Autodesk Inventor part; units mm, degrees
ref_plane "YZ Plane" through (0, 0, 0) normal (1, 0, 0) x (0, 1, 0)
ref_plane "XZ Plane" through (0, 0, 0) normal (0, 1, 0) x (-1, 0, 0)
ref_plane "XY Plane" through (0, 0, 0) normal (0, 0, 1) x (1, 0, 0)
sketch "Sketch1" plane through (0, 0, 0) normal (0, 0, 1) x (1, 0, 0)
  line L0 (-122.55, 8.89) -> (122.55, 8.89)
  line L1 (122.55, 8.89) -> (122.55, -8.89)
  line L2 (122.55, -8.89) -> (-122.55, -8.89)
  line L3 (-122.55, -8.89) -> (-122.55, 8.89)
  line L4 (-122.55, 8.89) -> (122.55, -8.89) construction
  line L5 (122.55, 8.89) -> (-122.55, -8.89) construction
  point P0 (0, 0)
  dimension "d0" = 245.1
  dimension "d1" = 17.78
extrude "Extrusion1" add sketch "Sketch1" along normal blind 6.2
fillet "Fillet1" radius 8.89 1 edges at (122.55, 8.89, 3.1)
fillet "Fillet2" radius 8.89 1 edges at (122.55, -8.89, 3.1)
fillet "Fillet3" radius 8.89 1 edges at (-122.55, -8.89, 3.1)
fillet "Fillet4" radius 8.89 1 edges at (-122.55, 8.89, 3.1)
sketch "Sketch6" plane through (0, 0, 0) normal (0, 0, -1) x (-1, 0, 0)
  circle A0 centre (111.8854, 0) radius 5.5644
  point P0 (0, 0)
extrude "Extrusion4" add sketch "Sketch6" along normal blind 7.2
sketch "Sketch7" plane through (0, 0, 0) normal (0, 0, -1) x (-1, 0, 0)
  point P0 (0, 0)
  point P1 (-112.5539, 0.8007)
hole "Hole3" at (112.5539, 0.8007, 0) direction (0, 0, 1) diameter 12.4257 end through all
equation "\"BendRadius\" = Thickness"
equation "\"BendReliefWidth\" = Thickness"
equation "\"BendReliefDepth\" = 0.5 * Thickness"
equation "\"CornerReliefSize\" = 4 * Thickness"
equation "\"MinimumRemnant\" = 2 * Thickness"
equation "\"TransitionRadius\" = BendRadius"
equation "\"JacobiRadiusSize\" = BendRadius"
equation "\"GapSize\" = Thickness"
properties part number "cranker rod part"
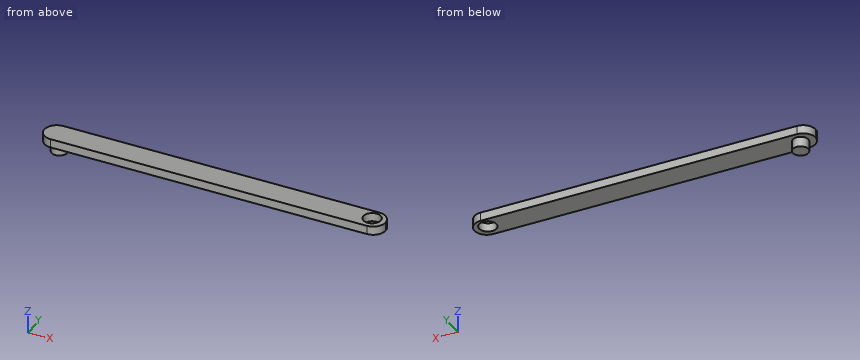
Part model, mm, in its own coordinate system. Round coordinates to 2 decimals unless told otherwise and drop trailing zeros. Write each loop counter-clockwise with the first axis right and the second up, starting at its lowest first coordinate (ties: lowest second). Pieces come first, ordered by that corner, then holes.
Item 1: Cut at A-A, the plane y = 3.5. Give the cut face in (x, z).
Results:
outline: (-121.83, 0) - (-116.21, 0) - (-116.21, -7.2) - (-107.56, -7.2) - (-107.56, 0) - (106.96, 0) - (106.96, 6.2) - (-121.83, 6.2) - close; (118.15, 0) - (121.83, 0) - (121.83, 6.2) - (118.15, 6.2) - close
Item 2: Cut at C-C, the plane x = -97. Give the cut face in (y, z), plus the area to 3 significant figures.
Results:
outline: (-8.89, 0) - (8.89, 0) - (8.89, 6.2) - (-8.89, 6.2) - close
area: 110 mm2
Item 3: Probe L1, parallel to Z at x = 70, y = 0.5; L2, parallel to X at y = 6.25, z = 2.25; L3, parallel to X at y = 2.5, z = 3. List the from-to ranges inside material, lowest first.
Results:
L1: z = 0 to 6.2
L2: x = -119.98 to 109.57, 115.54 to 119.98
L3: x = -122.19 to 106.58, 118.53 to 122.19
Item 4: Drop a flat-ended pin along its axis: pin 1 Ø9 at (x, y) = (-40, -0.5) entering from -Z. Give the stop position or say it passes through.
Results:
pin 1: stops at z = 0
